Work out the finished part from the listing and answer in its coordinate system (mm). A direction names the side the tool comes from. Round coordinates to 2 decimals unless told otherwise and drop trailing zeros. Order: outer loops, then holes, each group sorted by start corner. A loop starts at its lowest first (then second) coordinate and runs counter-clockwise, first axis right, second up. Notation, with made-up numbers: M -31,85.25 L 23,85.25 A8 cw 23,94.25 Z; hole C -10.75,5.5 d5. An arc over 180 degrees is marked long. Return JSON: item names as keys, results as strings.
from build123d import *

# Parameters (mm, degrees)
SKETCH1_W           = 125
SKETCH1_H           = 62
BOSS_EXTRUDE1_DEPTH = 12
BOSS_EXTRUDE5_DEPTH = 12
SKETCH6_R           = 7.5
CUT_EXTRUDE2_DEPTH  = 68
SKETCH8_W           = 12
SKETCH8_H           = 74
BOSS_EXTRUDE6_DEPTH = 15
SKETCH10_W          = 12
SKETCH10_H          = 50
BOSS_EXTRUDE7_DEPTH = 62
CUT_EXTRUDE3_DEPTH  = 62
SKETCH12_R          = 6
CUT_EXTRUDE4_DEPTH  = 62


with BuildPart() as part:
    # Sketch1 → Boss-Extrude1 (new body)
    with BuildSketch(Plane.XY):
        with Locations((48.885172376, -31)):
            Rectangle(SKETCH1_W, SKETCH1_H)
    extrude(amount=BOSS_EXTRUDE1_DEPTH)

    # Sketch5 → Boss-Extrude5 (add)
    with BuildSketch(Plane(origin=(0, 0, 0), x_dir=(1, 0, 0), z_dir=(0, 1, 0))):
        with BuildLine():
            Line((-3.819103259, 50), (101.180896741, 50))
            ThreePointArc((101.180896741, 50), (108.251964553, 47.071067812), (111.180896741, 40))
            Line((111.180896741, 40), (111.180896741, -24))
            Line((111.180896741, -24), (-13.819103259, -24))
            Line((-13.819103259, -24), (-13.819103259, 40))
            ThreePointArc((-13.819103259, 40), (-10.890171071, 47.071067812), (-3.819103259, 50))
        make_face()
    extrude(amount=BOSS_EXTRUDE5_DEPTH)

    # Sketch6 → Cut-Extrude2 (cut)
    with BuildSketch(Plane(origin=(0, 0, 0), x_dir=(-1, 0, 0), z_dir=(0, 0, -1))):
        with Locations((-96.385172376, -47)):
            Circle(SKETCH6_R)
        with Locations((-1.385172376, -15)):
            Circle(SKETCH6_R)
    extrude(amount=-CUT_EXTRUDE2_DEPTH, mode=Mode.SUBTRACT)

    # Sketch8 → Boss-Extrude6 (add)
    with BuildSketch(Plane(origin=(0, 12, 0), x_dir=(1, 0, 0), z_dir=(0, 1, 0))):
        with Locations((32.680896741, 13)):
            Rectangle(SKETCH8_W, SKETCH8_H)
        with Locations((64.680896741, 13)):
            Rectangle(SKETCH8_W, SKETCH8_H)
    extrude(amount=BOSS_EXTRUDE6_DEPTH)

    # Sketch10 → Boss-Extrude7 (add)
    with BuildSketch(Plane.XZ):
        with Locations((47.546562927, -25)):
            Rectangle(SKETCH10_W, SKETCH10_H)
    extrude(amount=BOSS_EXTRUDE7_DEPTH)

    # Sketch11 → Cut-Extrude3 (cut)
    with BuildSketch(Plane.ZY.offset(-41.546562927)):
        Polygon((-35.79571669, 0), (0, -62), (-50, -62), (-50, 0), align=None)
    extrude(amount=-CUT_EXTRUDE3_DEPTH, mode=Mode.SUBTRACT)

    # Sketch12 → Cut-Extrude4 (cut)
    with BuildSketch(Plane.XZ):
        with Locations(Location((6.180896741, -30, 0), (0, 0, 270))):
            Circle(SKETCH12_R)
        with Locations(Location((91.180896741, -20, 0), (0, 0, 270))):
            Circle(SKETCH12_R)
    extrude(amount=-CUT_EXTRUDE4_DEPTH, mode=Mode.SUBTRACT)


solid = part.part
Item 1: Find section B-B (z = 5.5). Determine the outline of the cut face in (x, y), plus the area to 3 significant figures.
Output:
{"outline": "M -13.82,0 L -13.61,0 L -13.61,-62 L 111.39,-62 L 111.39,0 L 111.18,0 L 111.18,12 L 70.68,12 L 70.68,27 L 58.68,27 L 58.68,12 L 38.68,12 L 38.68,27 L 26.68,27 L 26.68,12 L -13.82,12 Z; hole C 1.39,-15 d15; hole C 96.39,-47 d15", "area": "9,260 mm^2"}
Item 2: Find section A-A (y = 14). Determine the outline of the cut face in (x, z), plus the area to 3 significant figures.
Output:
{"outline": "M 26.68,-50 L 38.68,-50 L 38.68,24 L 26.68,24 Z; M 58.68,-50 L 70.68,-50 L 70.68,24 L 58.68,24 Z", "area": "1,780 mm^2"}
Item 3: Which of the six approach directions +Z, -Z, +X, -X, +Y, -Y give full straight-line access (tool end or side, diameter ignored) to faces 4 (the flat face through (63, 0, -22)), 5 (the flat face through (7, 12, -14)), 6 (the flat face through (58.681, 19, -12))?
Output:
{"face 4": "-Y", "face 5": "+Z, -Z, -X, +Y", "face 6": "+Z, -Z, +Y"}
Item 4: Each of these flat-tipped pins is pushed along its axis until it touches: pin 1 (8 mm diameter, centred on x = 0.5, z = 3.5, fed in from +Y); pin 2 (13 mm diameter, centred on y = -31.5, z = 5.5, fed in from -X); pin 3 (1 mm diameter, centred on x = 70, y = -51.5, fed in from -Z). Where does it stop, or does it pass through?
Output:
{"pin 1": "stops at y = 12", "pin 2": "stops at x = -13.61", "pin 3": "stops at z = 0"}
Item 5: The mould has two halves that part along Z. Classify faces 1 (the flat face through (82, -31, 0)), 2 (the cylindrical face through (85.86, 5.92, -22.77)), 3 (the cylindrical face through (3.01, -22.32, 5.92)): pulls with the +Z half, pulls with the -Z half, needs draft (parallel to the pull), parting line crosses it, or undercut.
Output:
{"face 1": "pulls with the -Z half", "face 2": "undercut", "face 3": "needs draft"}
Item 6: Find section D-D (z = -20). Determine the outline of the cut face in (x, y), plus the area to 3 significant figures.
Output:
{"outline": "M -13.82,0 L 41.55,0 L 41.55,-27.36 L 53.55,-27.36 L 53.55,0 L 85.18,0 L 85.18,12 L 70.68,12 L 70.68,27 L 58.68,27 L 58.68,12 L 38.68,12 L 38.68,27 L 26.68,27 L 26.68,12 L -13.82,12 Z; M 97.18,0 L 111.18,0 L 111.18,12 L 97.18,12 Z", "area": "2,040 mm^2"}
Item 7: Find section C-C (x = -1.5). Determine the outline of the cut face in (y, z).
Output:
{"outline": "M -62,0 L -21.92,0 L -21.92,12 L -62,12 Z; M -8.08,0 L 0,0 L 0,-50 L 12,-50 L 12,24 L 0,24 L 0,12 L -8.08,12 Z"}
Item 8: Consider line 1 along X through (y, z) = (8.5, -20); line 2 along X through (y, z) = (5, -30); line 3 along Z through (x, y) = (79, -31). Determine where each line is inside the solid, lowest interval first. Write a range as [from, to].
Output:
{"line 1": "x = [-13.82, 85.18], [97.18, 111.18]", "line 2": "x = [-13.82, 0.18], [12.18, 111.18]", "line 3": "z = [0, 12]"}
